from build123d import *

# Parameters (mm, degrees)
SKIZZE1_W                       = 200
SKIZZE1_H                       = 50
AUFSATZ_LINEAR_AUSTRAGEN1_DEPTH = 4
SKIZZE2_W                       = 15.5
SKIZZE2_H                       = 4
AUFSATZ_LINEAR_AUSTRAGEN2_DEPTH = 4
SCHNITT_LINEAR_AUSTRAGEN1_REACH = 6
SKIZZE4_W                       = 4
SKIZZE4_H                       = 15
SCHNITT_LINEAR_AUSTRAGEN2_REACH = 6
SKIZZE5_W                       = 3.7
SKIZZE5_H                       = 9.5
SCHNITT_LINEAR_AUSTRAGEN3_DEPTH = 4
SCHNITT_LINEAR_AUSTRAGEN4_REACH = 6
SKIZZE7_R                       = 8
SKIZZE7_R_2                     = 7


with BuildPart() as part:
    # Skizze1 → Aufsatz-Linear austragen1 (new body)
    with BuildSketch(Plane.XY):
        with Locations((100, 25)):
            Rectangle(SKIZZE1_W, SKIZZE1_H)
    extrude(amount=AUFSATZ_LINEAR_AUSTRAGEN1_DEPTH)

    # Skizze2 → Aufsatz-Linear austragen2 (add)
    with BuildSketch(Plane(origin=(0, 0, 4), x_dir=(-1, 0, 0), z_dir=(0, 0, -1))):
        with Locations((-174.8, -2)):
            Rectangle(SKIZZE2_W, SKIZZE2_H)
        with Locations((-124.8, -2)):
            Rectangle(SKIZZE2_W, SKIZZE2_H)
        with Locations((-74.8, -2)):
            Rectangle(SKIZZE2_W, SKIZZE2_H)
        with Locations((-24.8, -2)):
            Rectangle(SKIZZE2_W, SKIZZE2_H)
    extrude(amount=AUFSATZ_LINEAR_AUSTRAGEN2_DEPTH)

    # Skizze4 → Schnitt-Linear austragen1 (cut, up to next)
    with BuildSketch(Plane.XY.offset(4), mode=Mode.PRIVATE) as schnitt_linear_austragen1_sk1:
        with Locations((2, 25)):
            Rectangle(SKIZZE4_W, SKIZZE4_H)
    schnitt_linear_austragen1_tool1 = extrude(schnitt_linear_austragen1_sk1.sketch, amount=-SCHNITT_LINEAR_AUSTRAGEN1_REACH, mode=Mode.PRIVATE) & part.part
    add(schnitt_linear_austragen1_tool1.solids().sort_by_distance((2, 25, 4))[0], mode=Mode.SUBTRACT)
    # Skizze4 → Schnitt-Linear austragen1 (cut, up to next)
    with BuildSketch(Plane.XY.offset(4), mode=Mode.PRIVATE) as schnitt_linear_austragen1_sk2:
        with Locations((198, 25)):
            Rectangle(SKIZZE4_W, SKIZZE4_H)
    schnitt_linear_austragen1_tool2 = extrude(schnitt_linear_austragen1_sk2.sketch, amount=-SCHNITT_LINEAR_AUSTRAGEN1_REACH, mode=Mode.PRIVATE) & part.part
    add(schnitt_linear_austragen1_tool2.solids().sort_by_distance((198, 25, 4))[0], mode=Mode.SUBTRACT)

    # Skizze5 → Schnitt-Linear austragen2 (cut, up to next)
    with BuildSketch(Plane(origin=(0, 0, 0), x_dir=(-1, 0, 0), z_dir=(0, 0, -1)), mode=Mode.PRIVATE) as schnitt_linear_austragen2_sk1:
        with Locations((-100, 35.25)):
            Rectangle(SKIZZE5_W, SKIZZE5_H)
    schnitt_linear_austragen2_tool1 = extrude(schnitt_linear_austragen2_sk1.sketch, amount=-SCHNITT_LINEAR_AUSTRAGEN2_REACH, mode=Mode.PRIVATE) & part.part
    add(schnitt_linear_austragen2_tool1.solids().sort_by_distance((100, 35.25, 0))[0], mode=Mode.SUBTRACT)
    # Skizze5 → Schnitt-Linear austragen2 (cut, up to next)
    with BuildSketch(Plane(origin=(0, 0, 0), x_dir=(-1, 0, 0), z_dir=(0, 0, -1)), mode=Mode.PRIVATE) as schnitt_linear_austragen2_sk2:
        with Locations((-100, 15.75)):
            Rectangle(SKIZZE5_W, SKIZZE5_H)
    schnitt_linear_austragen2_tool2 = extrude(schnitt_linear_austragen2_sk2.sketch, amount=-SCHNITT_LINEAR_AUSTRAGEN2_REACH, mode=Mode.PRIVATE) & part.part
    add(schnitt_linear_austragen2_tool2.solids().sort_by_distance((100, 15.75, 0))[0], mode=Mode.SUBTRACT)

    # Skizze6 → Schnitt-Linear austragen3 (cut)
    with BuildSketch(Plane.XY.offset(4)):
        Polygon((52.05, 32.5), (48.05, 32.5), (48.05, 66.141635161), (-25.301318738, 66.141635161), (-25.301318738, -17.071359215), (48.05, -17.071359215), (48.05, 17.5), (52.05, 17.5), align=None)
    schnitt_linear_austragen3 = extrude(amount=-SCHNITT_LINEAR_AUSTRAGEN3_DEPTH, mode=Mode.SUBTRACT)

    # Spiegeln1: Schnitt-Linear austragen3 across plane
    add(schnitt_linear_austragen3.mirror(Plane.ZY.offset(-100)), mode=Mode.SUBTRACT)

    # Skizze7 → Schnitt-Linear austragen4 (cut, up to next)
    with BuildSketch(Plane.XY.offset(4), mode=Mode.PRIVATE) as schnitt_linear_austragen4_sk1:
        with Locations((125.855537029, 11.5)):
            Circle(SKIZZE7_R)
    schnitt_linear_austragen4_tool1 = extrude(schnitt_linear_austragen4_sk1.sketch, amount=-SCHNITT_LINEAR_AUSTRAGEN4_REACH, mode=Mode.PRIVATE) & part.part
    add(schnitt_linear_austragen4_tool1.solids().sort_by_distance((125.855537, 11.5, 4))[0], mode=Mode.SUBTRACT)
    # Skizze7 → Schnitt-Linear austragen4 (cut, up to next)
    with BuildSketch(Plane.XY.offset(4), mode=Mode.PRIVATE) as schnitt_linear_austragen4_sk2:
        with Locations((125.855537029, 38.5)):
            Circle(SKIZZE7_R)
    schnitt_linear_austragen4_tool2 = extrude(schnitt_linear_austragen4_sk2.sketch, amount=-SCHNITT_LINEAR_AUSTRAGEN4_REACH, mode=Mode.PRIVATE) & part.part
    add(schnitt_linear_austragen4_tool2.solids().sort_by_distance((125.855537, 38.5, 4))[0], mode=Mode.SUBTRACT)
    # Skizze7 → Schnitt-Linear austragen4 (cut, up to next)
    with BuildSketch(Plane.XY.offset(4), mode=Mode.PRIVATE) as schnitt_linear_austragen4_sk3:
        with Locations((74.842197302, 25)):
            Circle(SKIZZE7_R_2)
    schnitt_linear_austragen4_tool3 = extrude(schnitt_linear_austragen4_sk3.sketch, amount=-SCHNITT_LINEAR_AUSTRAGEN4_REACH, mode=Mode.PRIVATE) & part.part
    add(schnitt_linear_austragen4_tool3.solids().sort_by_distance((74.842197, 25, 4))[0], mode=Mode.SUBTRACT)
    # Skizze7 → Schnitt-Linear austragen4 (cut, up to next)
    with BuildSketch(Plane.XY.offset(4), mode=Mode.PRIVATE) as schnitt_linear_austragen4_sk4:
        with BuildLine():
            Line((120.354935265, 28.448963973), (120.354935265, 21.551036027))
            ThreePointArc((120.354935265, 21.551036027), (118.354935265, 19.551036027), (116.354935265, 21.551036027))
            Line((116.354935265, 21.551036027), (116.354935265, 28.448963973))
            ThreePointArc((116.354935265, 28.448963973), (118.354935265, 30.448963973), (120.354935265, 28.448963973))
        make_face()
    schnitt_linear_austragen4_tool4 = extrude(schnitt_linear_austragen4_sk4.sketch, amount=-SCHNITT_LINEAR_AUSTRAGEN4_REACH, mode=Mode.PRIVATE) & part.part
    add(schnitt_linear_austragen4_tool4.solids().sort_by_distance((118.354935, 25, 4))[0], mode=Mode.SUBTRACT)


solid = part.part
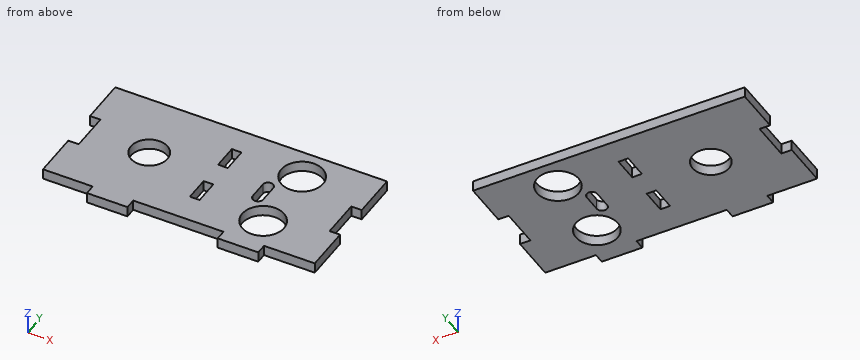
Read the model definition and answer for the solid it produces. Units are mm, in the model's axes. Give positions to 0.01 mm unless a question says otherwise; leave off trailing zeros. Loops run counter-clockwise (first coordinate to the right, second up) from the corner with the lowest first, then second, coordinate; pieces in that order, holes last. Notation, with made-up numbers: (28, 47) - (75, 47) arc R10 cw to (75, 60) - close; hole circle Ø8 at (-34.5, -15). An arc over 180 degrees is marked (long way). Answer as CSV lines item,"result". Start each with the question number.
1) Find section B-B (y = 7.5). Write down the section's boundary in (x, z), then the cut area to 3 significant figures.
2) Each of these flat-tipped pins is pushed along its axis until it touches: pin 1 Ø1.2 at (x, z) = (139, 2) entering from -Y; pin 2 Ø2 at (y, z) = (23, 1.5) entering from -X; pin 3 Ø1.2 at (y, z) = (25.5, 2) entering from +X. Where does it stop, or does it pass through?
3) Find section D-D (y = 38.5). Write down the section's boundary in (x, z), then the cut area to 3 significant figures.
4) Find section A-A (y = 25). Write down the section's boundary in (x, z), then the cut area to 3 significant figures.
5) Find section C-C (z = 2.6). State how many separate pieces and enclosed holes the cut face has, then the cut area to 3 significant figures.
6) Straight lines are drawn through the part: L1, parallel to X at y = 39, z = 3; L2, parallel to X at y = 22, z = 2.6; L3, parallel to Y at x = 128, z = 1.75. For each, find the intervals that lie inside material, in ascending order. Write a range as from..to.
Findings below:
1,outline,"(48.05, 0) - (118.93, 0) - (118.93, 4) - (48.05, 4) - close; (132.78, 0) - (151.95, 0) - (151.95, 4) - (132.78, 4) - close"
1,area,"360 mm^2"
2,pin 1,"y = 0"
2,pin 2,"x = 52.05"
2,pin 3,"x = 147.95"
3,outline,"(48.05, 0) - (98.15, 0) - (98.15, 4) - (48.05, 4) - close; (101.85, 0) - (117.86, 0) - (117.86, 4) - (101.85, 4) - close; (133.86, 0) - (151.95, 0) - (151.95, 4) - (133.86, 4) - close"
3,area,"337 mm^2"
4,outline,"(52.05, 0) - (67.84, 0) - (67.84, 4) - (52.05, 4) - close; (81.84, 0) - (116.35, 0) - (116.35, 4) - (81.84, 4) - close; (120.35, 0) - (147.95, 0) - (147.95, 4) - (120.35, 4) - close"
4,area,"312 mm^2"
5,separate pieces,"1"
5,enclosed holes,"6"
5,area,"4,530 mm^2"
6,L1,"48.05..98.15, 101.85..117.87, 133.84..151.95"
6,L2,"52.05..68.52, 81.17..116.35, 120.35..147.95"
6,L3,"-4..3.79, 19.21..30.79, 46.21..50"
